from build123d import *

# Parameters (mm, degrees)
F0_R     = 3.81
F1_DEPTH = 12.7


with BuildPart() as f1:
    # F0 (on Top) → F1 (new body)
    with BuildSketch(Plane.XY):
        Polygon((77.7875, 38.1), (77.7875, 142.875), (-77.7875, 142.875), (-77.7875, 71.4248), (-77.7875, 0), (-77.7875, -71.4248), (-77.7875, -142.875), (77.7875, -142.875), (77.7875, -38.1), (61.9125, -38.1), (61.9125, 38.1), align=None)
        with Locations((-65.0875, -84.1248)):
            Circle(F0_R, mode=Mode.SUBTRACT)
        with Locations((-65.0875, -58.7248)):
            Circle(F0_R, mode=Mode.SUBTRACT)
        with Locations((-65.0875, 58.7248)):
            Circle(F0_R, mode=Mode.SUBTRACT)
        with Locations((-65.0875, 84.1248)):
            Circle(F0_R, mode=Mode.SUBTRACT)
    extrude(amount=F1_DEPTH)


solid = f1.part
The model under review builds one solid part; all positions refer to its coordinate system, in mm. A direction names the side the tool comes from. Round coordinates to 2 decimals unless told otherwise and drop trailing zeros. Loops run counter-clockwise (first coordinate to the right, second up) from the corner with the lowest first, then second, coordinate; pieces in that order, holes last. Notation, with made-up numbers: (25, 44.5) -> (60, 44.5) arc R13 ccw to (60, 55.5) -> close; hole circle Ø7 at (38, 21.25). An arc over 180 degrees is marked (long way). Write item = value, one per line. Start each with the question number.
Item 1: Mouldability with a two-part tool opening along Y and no side actions: class faces 3 (the flat face through (-1, -142.875, 6)), 4 (the flat face through (-77.788, 2, 6)), 5 (the cylindrical face through (-61.568, 82.666, 6.261)) as released by +Y, released by -Y, zero draft, split by the parting line, or undercut.
Item 2: Take a section at B-B on z = 4.25. Give the boundary of the cut face in (x, y) (1 decimal).
Item 3: Take a section at C-C on y = -8. Give the boundary of the cut face in (x, z), plus the area to 3 significant figures.
Item 4: For faces 1 (the flat face through (1, 142.875, 6)), 2 (the flat face through (70, 38.1, 6)), list the 3-axis set-ups (+Z, -Z, +X, -X, +Y, -Y) from which the entire face can be reached by the end or side of a thin tool; tool diameter is ignored.
Item 5: To check wall thickness, follow L1, parallel to X at y = -84, z = 7.5; L2, parallel to Y at x = -62, z = 5 (3 decimals); L3, parallel to Y at x = -66.5, z = 6.5 (3 decimals). State the ranges of each line that lie inside material, in increasing order.
Item 6: Take a section at A-A on x = 66.5. Give the boundary of the cut face in (y, z) (3 decimals), plus the area to 3 significant figures.
Result:
q1.face_3 = released by -Y
q1.face_4 = zero draft
q1.face_5 = undercut
q2.outline = (-77.8, -142.9) -> (77.8, -142.9) -> (77.8, -38.1) -> (61.9, -38.1) -> (61.9, 38.1) -> (77.8, 38.1) -> (77.8, 142.9) -> (-77.8, 142.9) -> close; hole circle Ø7.6 at (-65.1, -84.1); hole circle Ø7.6 at (-65.1, -58.7); hole circle Ø7.6 at (-65.1, 58.7); hole circle Ø7.6 at (-65.1, 84.1)
q3.outline = (-77.79, 0) -> (61.91, 0) -> (61.91, 12.7) -> (-77.79, 12.7) -> close
q3.area = 1,770 mm²
q4.face_1 = +Z, -Z, +X, -X, +Y
q4.face_2 = +Z, -Z, +X
q5.L1 = -77.79 to -68.9, -61.28 to 77.79
q5.L2 = -142.875 to -86.357, -81.892 to -60.957, -56.492 to 56.492, 60.957 to 81.892, 86.357 to 142.875
q5.L3 = -142.875 to -87.663, -80.586 to -62.263, -55.186 to 55.186, 62.263 to 80.586, 87.663 to 142.875
q6.outline = (-142.875, 0) -> (-38.1, 0) -> (-38.1, 12.7) -> (-142.875, 12.7) -> close; (38.1, 0) -> (142.875, 0) -> (142.875, 12.7) -> (38.1, 12.7) -> close
q6.area = 2,660 mm²
